```python
from build123d import *

# Parameters (mm, degrees)
BOSS_EXTRUDE1_DEPTH = 381
SKETCH2_R           = 38.1
CUT_EXTRUDE1_DEPTH  = 889


with BuildPart() as part:
    # Sketch1 → Boss-Extrude1 (new body)
    with BuildSketch(Plane.XY):
        Polygon((0, 0), (9.525, 0), (9.525, 20.6248), (142.875, 20.6248), (142.875, 0), (152.4, 0), (152.4, 50.8), (142.875, 50.8), (142.875, 30.1752), (9.525, 30.1752), (9.525, 50.8), (0, 50.8), align=None)
    extrude(amount=-BOSS_EXTRUDE1_DEPTH)

    # Sketch2 → Cut-Extrude1 (cut)
    with BuildSketch(Plane(origin=(0, 30.1752, 0), x_dir=(-1, 0, 0), z_dir=(0, 1, 0))):
        with Locations((-76.2, -308.408066116)):
            Circle(SKETCH2_R)
        with Locations((-76.2, -190.5)):
            Circle(SKETCH2_R)
        with Locations(Location((-76.2, -72.591933884, 0), (0, 0, 270))):
            Circle(SKETCH2_R)
    extrude(amount=-CUT_EXTRUDE1_DEPTH, mode=Mode.SUBTRACT)


solid = part.part
```
The model under review builds one solid part; all positions refer to its coordinate system, in mm. A direction names the side the tool comes from. Round coordinates to 2 decimals unless told otherwise and drop trailing zeros. Write each loop counter-clockwise with the first axis right and the second up, starting at its lowest first coordinate (ties: lowest second). Pieces come first, ordered by that corner, then holes. Notation, with made-up numbers: M 48.25,19.5 L 60.25,19.5 A17 cw 60.25,48.5 Z; hole C 0,16.25 d1. An arc over 180 degrees is marked long. Use CSV: the item, a comma, the result in double quotes. Start each with the question number.
(1) Clearance check with a flat-ended pin moving along its axis: P1, Ø4, axis at x = 94, z = -38.5, coming from the +Y side. State where the tip first meets the part, or that it passes through.
(2) The part is to be moulded in two halves that separate along X. For faces 1 (the face through (152.4, 25, -188)), 2 (the face through (142.875, 41, -188)), 3 (the face through (148, 0, -188)), say which applies: +X half, -X half, draft (parallel to the pull), parting line (faces both ways), or undercut.
(3) We need section A-A, the plane z = -190.5. State the section outline as (x, y) points (3 decimals).
(4) For line 1 along Z through (x, y) = (76, 23); line 2 along X through (y, z) = (46.5, -80.5) (3 decimals); line 3 along Y through (x, z) = (28.5, -169), list the stretches that pass through material, from the lowest coordinate up.
(5) We need section D-D, the plane y = 24.5. State the section outline as (x, z) points.
(6) We need section B-B, the plane y = 41.5. State the section outline as (x, z) points (3 decimals), then the cut area to 3 significant figures.
(7) We need section C-C, the plane x = 76.2. State the section outline as (y, z) points.
(8) Tool access review of faces 4 (the face through (9.525, 40, -188)), 5 (the face through (148, 50.8, -188)), 6 (the face through (9.525, 10, -188)): name each direction out of +Z, -Z, +X, -X, +Y, -Y from which nothing blocks a thin tool from reaching the whole face with its end or side.
Findings:
1,P1,"y = 30.18"
2,face 1,"+X half"
2,face 2,"undercut"
2,face 3,"draft"
3,outline,"M 0,0 L 9.525,0 L 9.525,20.625 L 38.1,20.625 L 38.1,30.175 L 9.525,30.175 L 9.525,50.8 L 0,50.8 Z; M 114.3,20.625 L 142.875,20.625 L 142.875,0 L 152.4,0 L 152.4,50.8 L 142.875,50.8 L 142.875,30.175 L 114.3,30.175 Z"
4,line 1,"-381 to -346.51, -270.31 to -228.6, -152.4 to -110.69, -34.49 to 0"
4,line 2,"0 to 9.525, 142.875 to 152.4"
4,line 3,"20.62 to 30.18"
5,outline,"M 0,-381 L 152.4,-381 L 152.4,0 L 0,0 Z; hole C 76.2,-308.41 d76.2; hole C 76.2,-190.5 d76.2; hole C 76.2,-72.59 d76.2"
6,outline,"M 0,-381 L 9.525,-381 L 9.525,0 L 0,0 Z; M 142.875,-381 L 152.4,-381 L 152.4,0 L 142.875,0 Z"
6,area,"7,260 mm^2"
7,outline,"M 20.62,-381 L 30.18,-381 L 30.18,-346.51 L 20.62,-346.51 Z; M 20.62,-270.31 L 30.18,-270.31 L 30.18,-228.6 L 20.62,-228.6 Z; M 20.62,-152.4 L 30.18,-152.4 L 30.18,-110.69 L 20.62,-110.69 Z; M 20.62,-34.49 L 30.18,-34.49 L 30.18,0 L 20.62,0 Z"
8,face 4,"+Z, -Z, +Y"
8,face 5,"+Z, -Z, +X, -X, +Y"
8,face 6,"+Z, -Z, -Y"
